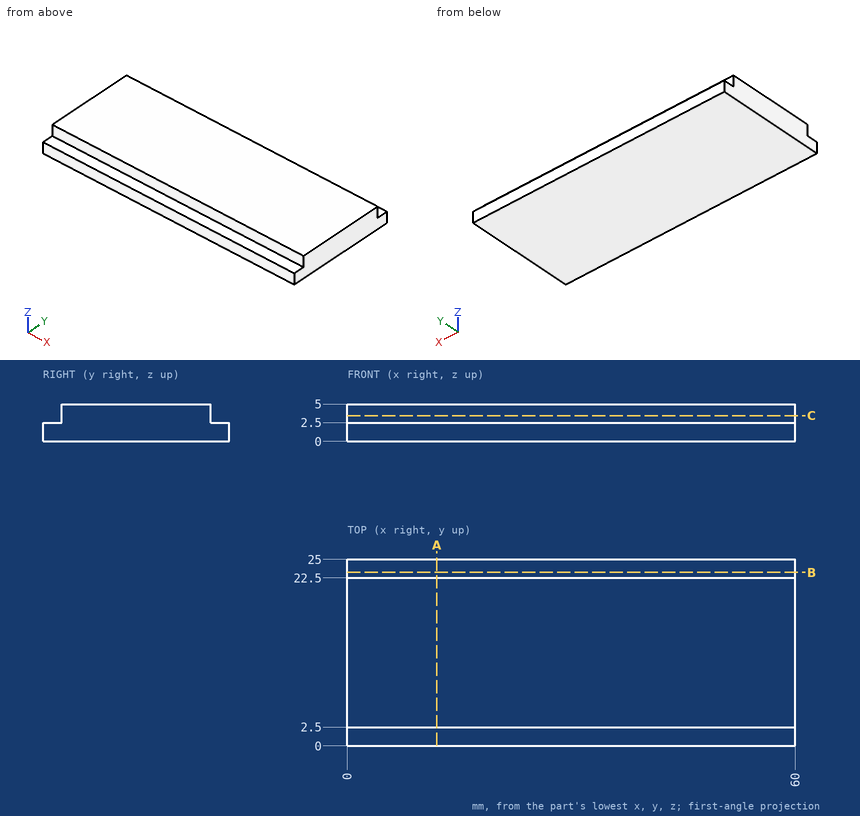
Part print with two shaded views. Sizes in mm from the minimum x, y, z corner. Coordinates: 2 decimals unless noted, no trailing zeros. Write each loop counter-clockwise with the first axis right and the second up, starting at its lowest first coordinate (ties: lowest second). Pieces come first, ordered by that corner, then holes. Notation, with made-up numbers: (21.5, -4.75) - (25.5, -4.75) arc R20 cw to (25.5, 20.25) - close; hole circle Ø5 at (74, -26.75). An arc over 180 degrees is marked (long way). One line per item, written item: value. Start each with the question number.
1. Slice it at B-B (y = 23.25). Write the cut outline in (x, z), plus the area to 3 significant figures.
2. Slice it at A-A (x = 12). Write the cut outline in (y, z), plus the area to 4 significant figures.
3. Slice it at C-C (z = 3.45). Write the cut outline in (x, y), plus the area to 3 significant figures.
4. Probe line 1 (Y direction, x = 34, z = 3.9); line 2 (Z direction, x = 33, y = 23). List the from-to ranges inside material, lowest first. Write a range as from..to.
5. Flat gauge pins, fed straight in: pin 1 (2 mm diameter, centred on x = 28, z = 4, fed in from -Y); pin 2 (6 mm diameter, centred on x = 44, y = 12, fed in from -Z); pin 3 (2 mm diameter, centred on x = 27, z = 4.5, fed in from +Y). Where does each tip first touch, or does it go through?
Answers below:
1. outline: (0, 0) - (60, 0) - (60, 2.5) - (0, 2.5) - close
1. area: 150 mm^2
2. outline: (0, 0) - (25, 0) - (25, 2.5) - (22.5, 2.5) - (22.5, 5) - (2.5, 5) - (2.5, 2.5) - (0, 2.5) - close
2. area: 112.5 mm^2
3. outline: (0, 2.5) - (60, 2.5) - (60, 22.5) - (0, 22.5) - close
3. area: 1,200 mm^2
4. line 1: y = 2.5..22.5
4. line 2: z = 0..2.5
5. pin 1: stops at y = 2.5
5. pin 2: stops at z = 0
5. pin 3: stops at y = 22.5
